The model under review builds one solid part; all positions refer to its coordinate system, in mm. A direction names the side the tool comes from. Coordinates: 2 decimals unless noted, no trailing zeros. Write each loop counter-clockwise with the first axis right and the second up, starting at its lowest first coordinate (ties: lowest second). Pieces come first, ordered by that corner, then holes. Notation, with made-up numbers: (3, 51.5) - (51, 51.5) arc R14 ccw to (51, 69.5) - close; hole circle Ø5 at (-1, 51). An arc over 180 degrees is marked (long way). Return JSON: item names as keys, results as strings. Group by question number.
(1) For pin 1 Ø10 at (x, z) = (9.5, 24.5) entering from +Y; pin 2 Ø3 at (x, z) = (8, 45.5) entering from +Y; pin 3 Ø6 at (x, z) = (-7, 1.5) entering from +Y; pin 4 Ø12 at (y, z) = (18, 34) entering from -X, all flat-tipped, find the tip position at first contact; note any pin that passes through.
(2) We need section A-A on z = 0. State the section outline as (x, y) points.
(3) Tool access review of faces 1 (the face through (0, 0, 0)), 2 (the face through (0, -1, -10)): name each direction out of +Z, -Z, +X, -X, +Y, -Y from which nothing blocks a thin tool from reaching the whole face with its end or side.
(4) We need section D-D on z = 14. State the section outline as (x, y) points, then the cut area to 3 significant figures.
(5) We need section B-B on x = -5. State the section outline as (y, z) points, then the cut area to 3 significant figures.
(6) We need section C-C on y = 13.5. State the section outline as (x, z) points, then the cut area to 3 significant figures.
(7) To check wall thickness, follow L1, parallel to X at y = -0.5, z = 0; L2, parallel to Y at x = -7, z = -1; L3, parallel to Y at x = -6, z = 24. State the ranges of each line that lie inside material, in increasing order. Write a range as from..to.
```python
from build123d import *

# Parameters (mm, degrees)
SKETCH1_W                    = 40
SKETCH1_H                    = 20
BASE_FLANGE1_DEPTH           = 1.5
SKETCH4_R                    = 2
CUT_EXTRUDE1_DEPTH           = 10
EDGE_FLANGE1_STRIP_CUT_DEPTH = 40
EDGE_FLANGE1_DEPTH           = 40
CHAMFER1_SIZE                = 5


# Sheet-metal steps are written as plain solids
with BuildPart() as part:
    # Sketch1 → Base-Flange1 (new body)
    with BuildSketch(Plane(origin=(0, 0, 0), x_dir=(1, 0, 0), z_dir=(0, 1, 0))):
        Rectangle(SKETCH1_W, SKETCH1_H)
    extrude(amount=-BASE_FLANGE1_DEPTH)

    # Sketch4 → Cut-Extrude1 (cut)
    with BuildSketch(Plane(origin=(0, 0, 0), x_dir=(1, 0, 0), z_dir=(0, 1, 0))):
        with Locations(Location((-12.349279575, 0, 0), (0, 0, 270))):
            Circle(SKETCH4_R)
        with Locations(Location((12.349279575, 0, 0), (0, 0, 270))):
            Circle(SKETCH4_R)
    extrude(amount=-CUT_EXTRUDE1_DEPTH, mode=Mode.SUBTRACT)

    # Edge-Flange1 strip (across the edge) → Edge-Flange1 strip cut (cut)
    with BuildSketch(Plane(origin=(-20, 0, 10), x_dir=(0, 0.9396926207859105, -0.3420201433256631), z_dir=(1, 0, 0))):
        Polygon((-4.397259152, 7.695663628), (-1.319077862, -0.761569959), (0.090461069, -0.248539744), (-2.987720221, 8.208693843), align=None)
    extrude(amount=EDGE_FLANGE1_STRIP_CUT_DEPTH, mode=Mode.SUBTRACT)

    # Edge-Flange1 section (across the edge) → Edge-Flange1 (add)
    with BuildSketch(Plane(origin=(-20, 0, 10), x_dir=(0, 0.9396926207859105, -0.3420201433256631), z_dir=(1, 0, 0))):
        with BuildLine():
            Line((-1.5, 0.264490471), (-1.5, 60))
            Line((-1.5, 60), (0, 60))
            Line((0, 60), (0, 0.264490471))
            ThreePointArc((0, 0.264490471), (0.02278837, 0.004018205), (0.090461069, -0.248539744))
            Line((0.090461069, -0.248539744), (-1.319077862, -0.761569959))
            ThreePointArc((-1.319077862, -0.761569959), (-1.454423259, -0.256454062), (-1.5, 0.264490471))
        make_face()
    extrude(amount=EDGE_FLANGE1_DEPTH)

    # Chamfer1
    chamfer1_edges = [part.edges().sort_by_distance(p)[0] for p in [
        (-20, 19.816439134, 66.638072355),
        (20, 19.816439134, 66.638072355),
        (-20, -0.75, -10),
        (20, -0.75, -10),
    ]]
    chamfer(chamfer1_edges, length=CHAMFER1_SIZE)


solid = part.part
```
Ans:
{
 "1": {"pin 1": "y = 7.1", "pin 2": "y = 13.47", "pin 3": "y = 0", "pin 4": "through"},
 "2": {"outline": "(-20, -1.5) - (-14.35, -1.5) - (-14.35, 0) - (-20, 0) - close; (-10.35, -1.5) - (10.35, -1.5) - (10.35, 0) - (-10.35, 0) - close; (14.35, -1.5) - (20, -1.5) - (20, 0) - (14.35, 0) - close"},
 "3": {"face 1": "-Z, +X, -X, +Y", "face 2": "-Z, +X, -X, +Y, -Y"},
 "4": {"outline": "(-20, -0.14) - (20, -0.14) - (20, 1.46) - (-20, 1.46) - close", "area": "63.9 mm²"},
 "5": {"outline": "(-1.5, -10) - (0, -10) - (0, 9.74) arc R1.5 cw to (0.09, 10.25) - (20.52, 66.38) - (19.11, 66.89) - (-1.32, 10.76) arc R3 ccw to (-1.5, 9.74) - close", "area": "120 mm²"},
 "6": {"outline": "(-20, 47.09) - (20, 47.09) - (20, 51.48) - (-20, 51.48) - close", "area": "175 mm²"},
 "7": {"L1": "-20..-14.35, -10.35..10.35, 14.35..20", "L2": "-1.5..0", "L3": "3.5..5.1"}
}
